Can you work these out from the model? Positions are in its coordinate system, mm. Give positions to 0.01 mm unless a question says otherwise; leave off trailing zeros. Answer in a Markdown table with one row per item.
from build123d import *

# Parameters (mm, degrees)
F1_DEPTH = 7.62
F2_R     = 7.61999


# Not quite as in the source:
# - a fillet or chamfer is up to 0.001 mm smaller than in the source, because OpenCascade refuses the exact size


with BuildPart() as f1:
    # F0 (on Top) → F1 (new body)
    with BuildSketch(Plane.XY):
        with BuildLine():
            ThreePointArc((64.2620003332, -67.437), (131.6990003332, 0), (64.2620003332, 67.437))
            Line((64.2620003332, 67.437), (-64.2620003332, 67.437))
            ThreePointArc((-64.2620003332, 67.437), (-131.6990003332, 0), (-64.2620003332, -67.437))
            Line((-64.2620003332, -67.437), (64.2620003332, -67.437))
        make_face()
        with BuildLine():
            Line((-64.2620003332, 54.737), (64.2620003332, 54.737))
            ThreePointArc((64.2620003332, 54.737), (118.9990003332, 0), (64.2620003332, -54.737))
            Line((64.2620003332, -54.737), (-64.2620003332, -54.737))
            ThreePointArc((-64.2620003332, -54.737), (-118.9990003332, 0), (-64.2620003332, 54.737))
        make_face(mode=Mode.SUBTRACT)
        with BuildLine():
            ThreePointArc((64.2620003332, -54.737), (9.5250003332, 0), (64.2620003332, 54.737))
            Line((64.2620003332, 54.737), (-64.2620003332, 54.737))
            ThreePointArc((-64.2620003332, 54.737), (-9.5250003332, 0), (-64.2620003332, -54.737))
            Line((-64.2620003332, -54.737), (64.2620003332, -54.737))
        make_face()
    extrude(amount=F1_DEPTH)

    # F2 (radius 7.62 in the source; OpenCascade refuses exactly that, so slightly less here)
    f2_edges = [f1.edges().sort_by_distance(p)[0] for p in [
        (-131.699, 0, 7.62),
    ]]
    fillet(f2_edges, radius=F2_R)


solid = f1.part
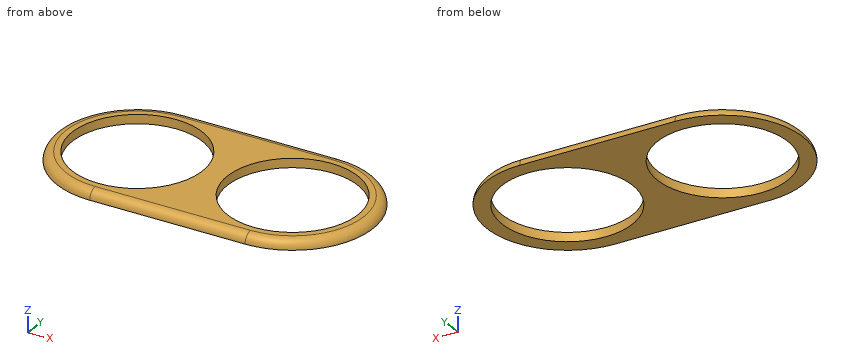
Q1. For pin 1 (3 mm diameter, centred on x = 46.5, z = 3.5, fed in from +Y); pin 2 (4 mm diameter, centred on y = -18, z = 6, fed in from -X); pin 3 (4 mm diameter, centred on y = -37, z = 2.5, fed in from +X), each with a flat end and sliding along its axis, tell me the tip position at first contact or that it passes through.
Checked values:
| item | result |
|---|---|
| pin 1 | stops at y = 67.17 |
| pin 2 | stops at x = -128.19 |
| pin 3 | stops at x = 121.58 |
Q2. Imagine slicing it at B-B, the plane y = 0. Count the separate pieces of the cut face and the enclosed holes in it, and give its area (3 significant figures).
Checked values:
| item | result |
|---|---|
| separate pieces | 3 |
| enclosed holes | 0 |
| area | 314 mm² |
Q3. If I drill on line 1 (X direction, y = 34, z = 5); line 2 (X direction, y = -14, z = 5.25); line 3 (Y direction, x = 21, z = 1.25), over which ranges is the centre line in solid material (lowest first)? Write a range as [from, to].
Checked values:
| item | result |
|---|---|
| line 1 | x = [-120.32, -107.16], [-21.37, 21.37], [107.16, 120.32] |
| line 2 | x = [-128.08, -117.18], [-11.35, 11.35], [117.18, 128.08] |
| line 3 | y = [-67.33, -33.53], [33.53, 67.33] |
